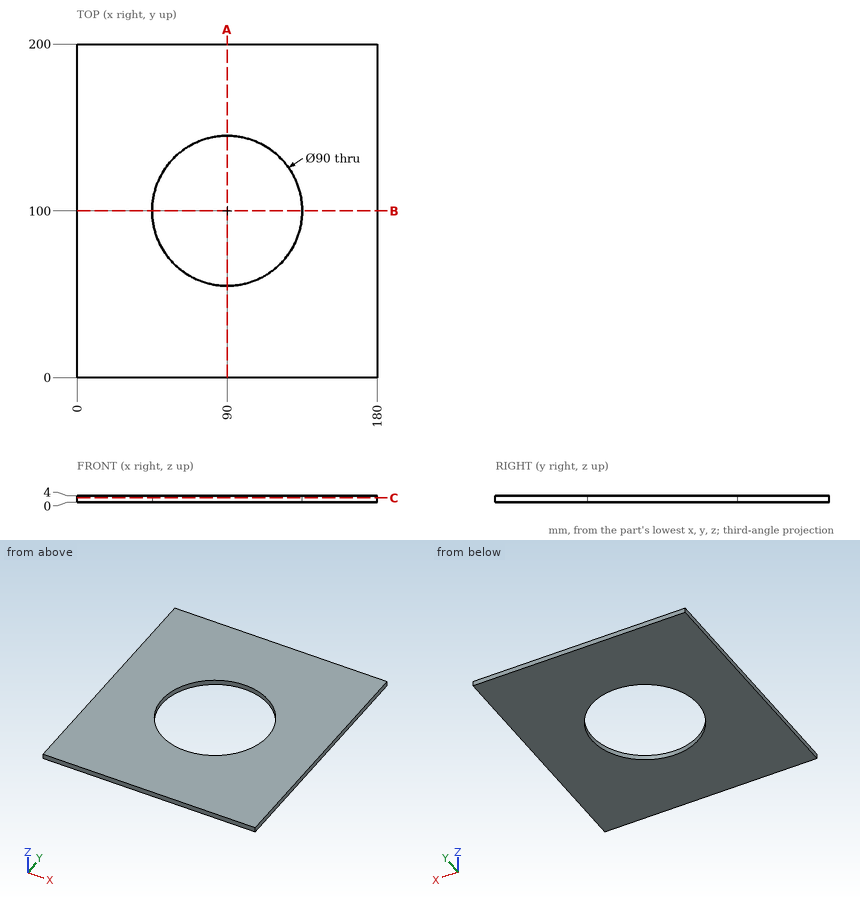
Geometry: see drawing. Coordinates: mm, zero at the bounding-box minimum. Give positions to 0.01 mm unless a question says otherwise; leave off trailing zeros. Loops run counter-clockwise (first coordinate to the right, second up) from the corner with the lowest first, then second, coordinate; pieces in that order, holes last. Notation, with made-up numbers: (36, 60.25) - (74, 60.25) arc R22 ccw to (74, 91.25) - close; hole circle Ø11 at (6.5, -18.5). An arc over 180 degrees is marked (long way). Use CSV: the item, a comma, the result in double quotes.
1) Cut plane C-C (z = 2.7). Output: boundary loops of the cut face in (x, y).
Worked out:
outline,"(0, 0) - (180, 0) - (180, 200) - (0, 200) - close; hole circle Ø90 at (90, 100)"
2) Cut plane B-B (y = 100). Output: boundary loops of the cut face in (x, z).
Worked out:
outline,"(0, 0) - (45, 0) - (45, 4) - (0, 4) - close; (135, 0) - (180, 0) - (180, 4) - (135, 4) - close"
3) Cut plane A-A (x = 90). Output: boundary loops of the cut face in (y, z).
Worked out:
outline,"(0, 0) - (55, 0) - (55, 4) - (0, 4) - close; (145, 0) - (200, 0) - (200, 4) - (145, 4) - close"
4) Line query: line 1 (X direction, y = 100, z = 3.05); line 2 (Y direction, x = 90, z = 2); line 3 (X direction, y = 63, z = 1.3). Output: solid intervals per line, ascending.
Worked out:
line 1,"x = 0 to 45, 135 to 180"
line 2,"y = 0 to 55, 145 to 200"
line 3,"x = 0 to 64.39, 115.61 to 180"
